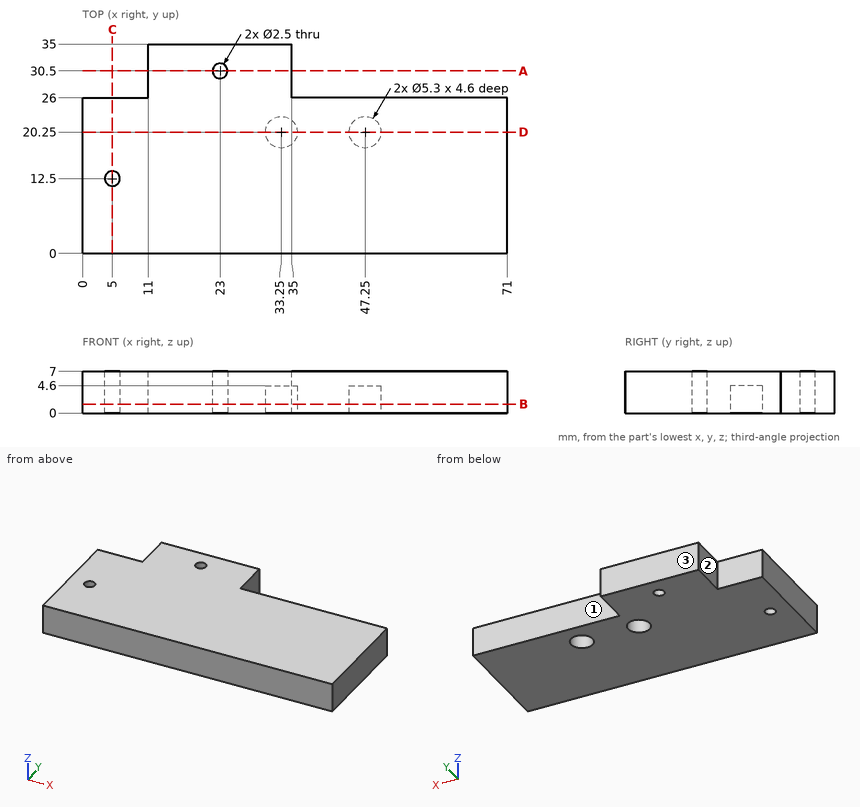
Verification items for this drawing (mm, ordinates from the low corner). A direction names the side the tool comes from. Coordinates: 2 decimals unless noted, no trailing zeros. Order: outer loops, then holes, each group sorted by start corner. A loop starts at its lowest first (then second) coordinate and runs counter-clockwise, first axis right, second up. Notation, with made-up numbers: (25, 2.25) -> (64, 2.25) arc R9 ccw to (64, 18.25) -> close; hole circle Ø11 at (67.25, 29). An arc over 180 degrees is marked (long way). Put each result on its own line as item: value. Start each with the question number.
1. Go/stop test with flat-tipped pins: pin 1 Ø3 at (x, y) = (23, 30.5) entering from +Z; pin 2 Ø3.5 at (y, z) = (30.5, 3) entering from -X; pin 3 Ø3.5 at (x, z) = (7, 4.5) entering from +Y; pin 4 Ø3 at (x, y) = (47.25, 20.25) entering from -Z. Record where each tip stops, or that it passes through.
2. Cross-section at A-A, the plane y = 30.5. Record the boundary of the cut face in (x, z).
3. Cross-section at B-B, the plane z = 1.5. Record the boundary of the cut face in (x, y).
4. Material ranges on L1, parallel to X at y = 21, z = 3.75; L2, parallel to Y at x = 33.25, z = 2.15; L3, parallel to Y at x = 10, z = 2, recorded low to high. Write a range as [from, to].
5. Cross-section at C-C, the plane x = 5. Record the boundary of the cut face in (y, z), then the cut area to 4 significant figures.
6. Cross-section at D-D, the plane y = 20.25. Record the boundary of the cut face in (x, z).
7. Access from +Z, -Z, +X, -X, +Y, -Y to the whole of each face (thin tool, end or side, straight path). Record for the marked faces 1, 2 and 3.
Computed:
1. pin 1: z = 7
1. pin 2: x = 11
1. pin 3: y = 26
1. pin 4: z = 4.6
2. outline: (11, 0) -> (21.75, 0) -> (21.75, 7) -> (11, 7) -> close; (24.25, 0) -> (35, 0) -> (35, 7) -> (24.25, 7) -> close
3. outline: (0, 0) -> (71, 0) -> (71, 26) -> (35, 26) -> (35, 35) -> (11, 35) -> (11, 26) -> (0, 26) -> close; hole circle Ø2.5 at (5, 12.5); hole circle Ø2.5 at (23, 30.5); hole circle Ø5.3 at (33.25, 20.25); hole circle Ø5.3 at (47.25, 20.25)
4. L1: [0, 30.71], [35.79, 44.71], [49.79, 71]
4. L2: [0, 17.6], [22.9, 35]
4. L3: [0, 26]
5. outline: (0, 0) -> (11.25, 0) -> (11.25, 7) -> (0, 7) -> close; (13.75, 0) -> (26, 0) -> (26, 7) -> (13.75, 7) -> close
5. area: 164.5 mm2
6. outline: (0, 0) -> (30.6, 0) -> (30.6, 4.6) -> (35.9, 4.6) -> (35.9, 0) -> (44.6, 0) -> (44.6, 4.6) -> (49.9, 4.6) -> (49.9, 0) -> (71, 0) -> (71, 7) -> (0, 7) -> close
7. face 1: +Z, -Z, +X, +Y
7. face 2: +Z, -Z, -X, +Y
7. face 3: +Z, -Z, +X, -X, +Y
